Here's how the part is built. I have some questions about the finished solid (model axes, mm). A direction names the side the tool comes from. Round coordinates to 2 decimals unless told otherwise and drop trailing zeros. Write each loop counter-clockwise with the first axis right and the second up, starting at its lowest first coordinate (ties: lowest second). Pieces come first, ordered by that corner, then holes. Notation, with made-up numbers: (51.5, 5) -> (104.5, 5) arc R24 cw to (104.5, 25) -> close; hole circle Ø8 at (-12, 77.5). An arc over 180 degrees is marked (long way). Answer as CSV lines item,"result".
Autodesk Inventor part; units mm, degrees
ref_plane "YZ Plane" through (0, 0, 0) normal (1, 0, 0) x (0, 1, 0)
ref_plane "XZ Plane" through (0, 0, 0) normal (0, 1, 0) x (-1, 0, 0)
ref_plane "XY Plane" through (0, 0, 0) normal (0, 0, 1) x (1, 0, 0)
sketch "Schizzo1" plane through (0, 0, 0) normal (0, 0, 1) x (1, 0, 0)
  circle A0 centre (0, 0) radius 5
  line L0 (2.8868, 5) -> (5.7735, 0)
  line L1 (5.7735, 0) -> (2.8868, -5)
  line L2 (2.8868, -5) -> (-2.8868, -5)
  line L3 (-2.8868, -5) -> (-5.7735, 0)
  line L4 (-5.7735, 0) -> (-2.8868, 5)
  line L5 (-2.8868, 5) -> (2.8868, 5)
  point P0 (0, 5)
  dimension "d0" = 10
extrude "Estrusione1" add sketch "Schizzo1" along normal blind 4
sketch "Schizzo3" plane through (0, 0, 0) normal (0, 0, -1) x (-1, 0, 0)
  circle A0 centre (0, 0) radius 3
  dimension "d3" = 6
extrude "Estrusione2" add sketch "Schizzo3" along normal blind 100
thread "Filettatura1"
fillet "Raccordo1" radius 1 1 edges at (3, 0, -100)
properties part number "18_Vite_M6_L100"
1. Suppose I cut it at A-A on x = 0. Please give me the cut outline in (y, z), and give its area (3 significant figures).
Numbers:
outline,"(-5, 0) -> (-3, 0) -> (-3, -99) arc R1 ccw to (-2, -100) -> (2, -100) arc R1 ccw to (3, -99) -> (3, 0) -> (5, 0) -> (5, 4) -> (-5, 4) -> close"
area,"640 mm^2"
2. For pin 1 Ø1.5 at (y, z) = (3.5, -63.5) entering from -X, with a flat end and sliding along its axis, tell me the tip position at first contact or that it passes through.
Numbers:
pin 1,"stops at x = -1.2"
3. Suppose I cut it at D-D on x = -4.5. Please give me the cut outline in (y, z), and give its area (3 significant figures).
Numbers:
outline,"(-2.21, 0) -> (2.21, 0) -> (2.21, 4) -> (-2.21, 4) -> close"
area,"17.6 mm^2"
4. On a 3-axis mill with a long thin cutter (end or side, diameter ignored), from which of +Z, -Z, +X, -X, +Y, -Y can I reach the whole of each face in a straight line? I mean faces 1 (the face through (3, 0, -49)), 2 (the face through (4.31, 2.535, 1.972)). Say none if no direction works.
Numbers:
face 1,"-Z"
face 2,"+Z, -Z, +X, +Y"
5. Suppose I cut it at C-C on y = -4. Please give me the cut outline in (x, z), and give its area (3 significant figures).
Numbers:
outline,"(-3.46, 0) -> (3.46, 0) -> (3.46, 4) -> (-3.46, 4) -> close"
area,"27.7 mm^2"
6. Suppose I cut it at B-B on z = -91. Please give me the cut outline in (x, y).
Numbers:
outline,"circle Ø6 at (0, 0)"
7. If I drill on line 1 (Z direction, x = -1.5, y = 4); line 2 (Y direction, x = -2.25, z = -26); line 3 (Y direction, x = 0, z = -79), over which ranges is the centre line in solid material (lowest first)?
Numbers:
line 1,"z = 0 to 4"
line 2,"y = -1.98 to 1.98"
line 3,"y = -3 to 3"
